Part print with two shaded views. Sizes in mm from the minimum x, y, z corner. A direction names the side the tool comes from. Round coordinates to 2 decimals unless told otherwise and drop trailing zeros. Write each loop counter-clockwise with the first axis right and the second up, starting at its lowest first coordinate (ties: lowest second). Pieces come first, ordered by that corner, then holes. Notation, with made-up numbers: (-16.5, -20) -> (34.5, -20) arc R34 cw to (34.5, 13) -> close; hole circle Ø9 at (76.5, 86). An arc over 180 degrees is marked (long way). Put each result on its own line as item: value. Start each with the question number.
1. Saw through at D-D on z = 43. List the corners of the cut face in (x, y), and give its area (3 significant figures).
2. Saw through at C-C on z = 23.5. List the corners of the cut face in (x, y), and give its area (3 significant figures).
3. Drill centre lines: line 1 (Z direction, x = 23, y = 28); line 2 (X direction, y = 18.25, z = 23.5); line 3 (X direction, y = 26, z = 7). Where is each one in solid material? Low to high. Write a range as from..to.
4. 3-axis set-ups, long thin cutter, end or side, ignore diameter. For the marked faces 5 and 6: which of +Z, -Z, +X, -X, +Y, -Y reach the whole face in a straight line?
5. Flat gauge pins, fed straight in: P1, Ø4, axis at x = 23, z = 23.5, coming from the +Y side; P2, Ø6.5, axis at x = 7, z = 7, coming from the -Y side; P3, Ø4, axis at y = 15, z = 43, coming from the +X side. Where does each tip first touch, or does it go through?
6. Saw through at A-A on x = 7. List the corners of the cut face in (y, z).
7. Saw through at B-B on y = 21.5. List the corners of the cut face in (x, z).
8. Pull direction X, two halves, no side cores. Call the marked faces 1, 2, 3 and 4: pulls with the +X half, pulls with the -X half, needs draft (parallel to the pull), parting line crosses it, or undercut.
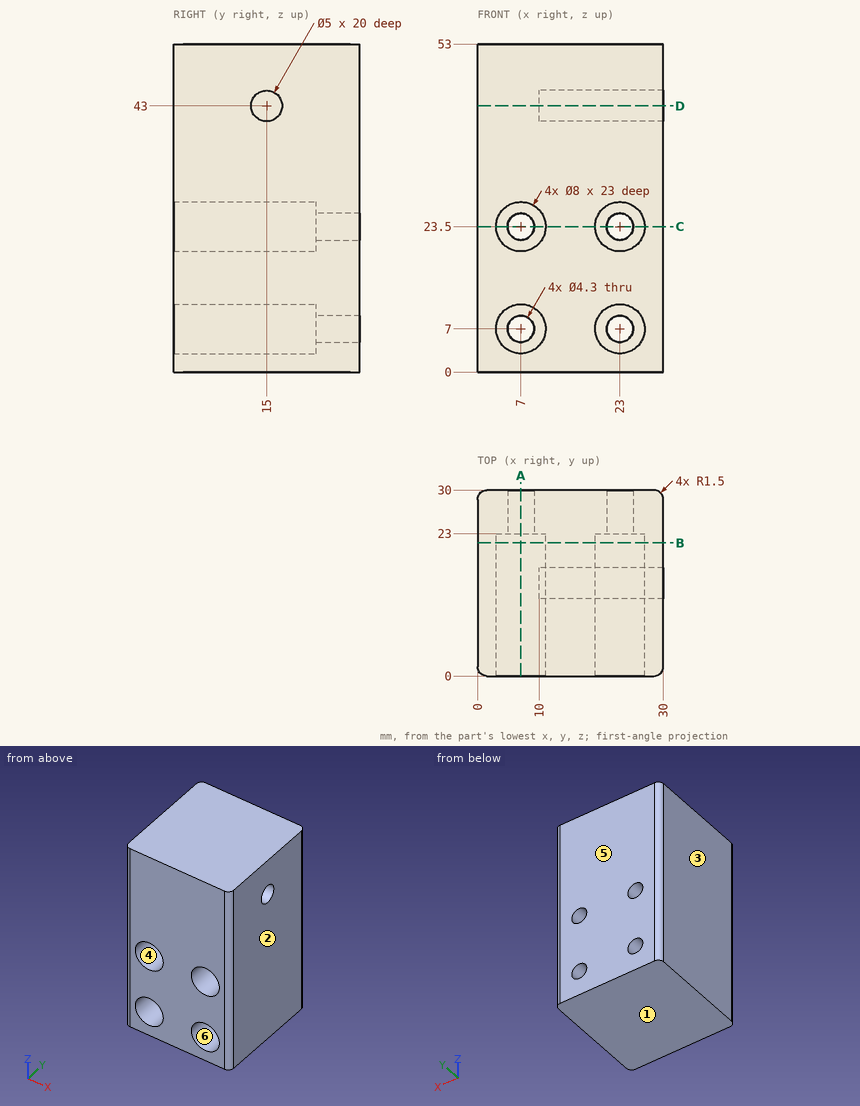
Return value:
1. outline: (0, 1.5) arc R1.5 ccw to (1.5, 0) -> (28.5, 0) arc R1.5 ccw to (30, 1.5) -> (30, 12.5) -> (10, 12.5) -> (10, 17.5) -> (30, 17.5) -> (30, 28.5) arc R1.5 ccw to (28.5, 30) -> (1.5, 30) arc R1.5 ccw to (0, 28.5) -> close
1. area: 798 mm^2
2. outline: (0, 1.5) arc R1.5 ccw to (1.5, 0) -> (3, 0) -> (3, 23) -> (4.85, 23) -> (4.85, 30) -> (1.5, 30) arc R1.5 ccw to (0, 28.5) -> close; (9.15, 23) -> (11, 23) -> (11, 0) -> (19, 0) -> (19, 23) -> (20.85, 23) -> (20.85, 30) -> (9.15, 30) -> close; (25.15, 23) -> (27, 23) -> (27, 0) -> (28.5, 0) arc R1.5 ccw to (30, 1.5) -> (30, 28.5) arc R1.5 ccw to (28.5, 30) -> (25.15, 30) -> close
2. area: 470 mm^2
3. line 1: z = 0..4.85, 9.15..21.35, 25.65..53
3. line 2: x = 0..3, 11..19, 27..30
3. line 3: x = 0..4.85, 9.15..20.85, 25.15..30
4. face 5: +Z, -Z, +X, -X, +Y
4. face 6: -Y
5. P1: passes through
5. P2: stops at y = 23
5. P3: stops at x = 10
6. outline: (0, 0) -> (30, 0) -> (30, 4.85) -> (23, 4.85) -> (23, 3) -> (0, 3) -> close; (0, 11) -> (23, 11) -> (23, 9.15) -> (30, 9.15) -> (30, 21.35) -> (23, 21.35) -> (23, 19.5) -> (0, 19.5) -> close; (0, 27.5) -> (23, 27.5) -> (23, 25.65) -> (30, 25.65) -> (30, 53) -> (0, 53) -> close
7. outline: (0, 0) -> (30, 0) -> (30, 53) -> (0, 53) -> close; hole circle Ø8 at (7, 7); hole circle Ø8 at (7, 23.5); hole circle Ø8 at (23, 7); hole circle Ø8 at (23, 23.5)
8. face 1: needs draft
8. face 2: pulls with the +X half
8. face 3: pulls with the -X half
8. face 4: undercut
